from build123d import *

# Parameters (mm, degrees)
F0_W     = 38.1
F0_H     = 38.1
F1_DEPTH = 25.4
F3_R     = 6.35
F4_DEPTH = 25.4
F7_D     = 10.16


with BuildPart() as f1:
    # F0 (on Top) → F1 (new body)
    with BuildSketch(Plane.XY):
        with Locations((19.05, 19.05)):
            Rectangle(F0_W, F0_H)
    extrude(amount=F1_DEPTH)

    # F3 (on offset) → F4 (join)
    with BuildSketch(Plane.XY.offset(25.4)):
        with Locations((19.05, 19.05)):
            Circle(F3_R)
    extrude(amount=F4_DEPTH)

    # F7 (through all)
    with Locations(Plane.XY.offset(50.8)):
        with Locations((19.05, 19.05)):
            Hole(F7_D / 2)


solid = f1.part
Geometry check sheet. Reference: the model listing, model coordinates, mm. A direction names the side the tool comes from. Give positions to 0.01 mm unless a question says otherwise; leave off trailing zeros. Loops run counter-clockwise (first coordinate to the right, second up) from the corner with the lowest first, then second, coordinate; pieces in that order, holes last. Notation, with made-up numbers: M 43,42 L 95,42 A17 cw 95,71 Z; hole C 30.5,22 d1. An arc over 180 degrees is marked long. Write each question's results on one line, items separated by ' | '.
1) Thickness scan on line 1 (X direction, y = 19, z = 38); line 2 (Y direction, x = 19.05, z = 11). Record the ranges inside material, lowest first.
Answers follow:
line 1: 12.7 to 13.97, 24.13 to 25.4 | line 2: 0 to 13.97, 24.13 to 38.1
2) Gauge pin test, flat ends, axial feed: pin 1 (8 mm diameter, centred on x = 10, z = 35.5, fed in from +Y); pin 2 (10 mm diameter, centred on x = 11.5, z = 45, fed in from +Y); pin 3 (6 mm diameter, centred on x = 11.5, y = 29.5, fed in from +Z). Record the tip position at first contact, or that the pin passes through.
Answers follow:
pin 1: y = 22.9 | pin 2: y = 24.87 | pin 3: z = 25.4
3) Tool access check on faces 1 (the face through (19, 28, 25.4)), 2 (the face through (19, 38.1, 13)). Record the directions out of +Z, -Z, +X, -X, +Y, -Y that give a thin tool (end or side, any length) a straight path to the whole face; none if there is none.
Answers follow:
face 1: +Z | face 2: +Z, -Z, +X, -X, +Y
4) Section check D-D, the plane y = 8. Record the boundary of the cut face in (x, z).
Answers follow:
outline: M 0,0 L 38.1,0 L 38.1,25.4 L 0,25.4 Z
5) Section check C-C, the plane z = 19. Record the boundary of the cut face in (x, y).
Answers follow:
outline: M 0,0 L 38.1,0 L 38.1,38.1 L 0,38.1 Z; hole C 19.05,19.05 d10.16
6) Section check A-A, the plane x = 19.05. Record the boundary of the cut face in (y, z).
Answers follow:
outline: M 0,0 L 13.97,0 L 13.97,50.8 L 12.7,50.8 L 12.7,25.4 L 0,25.4 Z; M 24.13,0 L 38.1,0 L 38.1,25.4 L 25.4,25.4 L 25.4,50.8 L 24.13,50.8 Z
